For this review, take the finished solid that the model builds, in its own axes (mm). A direction names the side the tool comes from. Give positions to 0.01 mm unless a question says otherwise; leave off trailing zeros. Loops run counter-clockwise (first coordinate to the right, second up) from the corner with the lowest first, then second, coordinate; pieces in that order, holes last. Notation, with made-up numbers: (85.25, 15.25) - (124.25, 15.25) arc R8 cw to (124.25, 20.25) - close; hole circle Ø9 at (-33, 43.25). An arc over 180 degrees is marked (long way). Answer in a Markdown table with one row per item.
```python
from build123d import *

# Parameters (mm, degrees)
BOSS_EXTRUDE1_DEPTH        = 6
SKETCH2_R                  = 2.025
CUT_EXTRUDE1_DEPTH         = 68.55671766
SKETCH3_R                  = 2
CUT_EXTRUDE2_DEPTH         = 67.962004906
FILLET1_R                  = 5
M3X0_5_TAPPED_HOLE1_REACH  = 72.92
M3X0_5_TAPPED_HOLE1_BORE_R = 1.5


with BuildPart() as part:
    # Sketch1 → Boss-Extrude1 (new, symmetric)
    with BuildSketch(Plane.XY):
        Polygon((4, 0), (-23, 0), (-35, -8), (-66.211102551, -8), (-66.211102551, -4), (-36.211102551, -4), (-24.211102551, 4), (4, 4), align=None)
    extrude(amount=BOSS_EXTRUDE1_DEPTH, both=True)

    # Sketch2 → Cut-Extrude1 (cut, through all)
    with BuildSketch(Plane(origin=(0, 4, 0), x_dir=(1, 0, 0), z_dir=(0, 1, 0))):
        with Locations(Location((0, 0, 0), (0, 0, 180))):
            Circle(SKETCH2_R)
    extrude(amount=-CUT_EXTRUDE1_DEPTH, mode=Mode.SUBTRACT)

    # Sketch3 → Cut-Extrude2 (cut, through all)
    with BuildSketch(Plane(origin=(0, -4, 0), x_dir=(1, 0, 0), z_dir=(0, 1, 0))):
        with Locations(Location((-62.211102551, 0, 0), (0, 0, 270))):
            Circle(SKETCH3_R)
        with Locations(Location((-52.211102551, 2, 0), (0, 0, 270))):
            Circle(SKETCH3_R)
        with Locations(Location((-42.211102551, -2, 0), (0, 0, 270))):
            Circle(SKETCH3_R)
    extrude(amount=-CUT_EXTRUDE2_DEPTH, mode=Mode.SUBTRACT)

    # Fillet1
    fillet1_edges = [part.edges().sort_by_distance(p)[0] for p in [
        (4, 2, -6),
        (-23, 0, 0),
        (-35, -8, 0),
        (-36.211102551, -4, 0),
        (-24.211102551, 4, 0),
        (-66.211102551, -6, 6),
        (4, 2, 6),
        (-66.211102551, -6, -6),
    ]]
    fillet(fillet1_edges, radius=FILLET1_R)

    # M3x0.5 Tapped Hole1 bore → M3x0.5 Tapped Hole1 (cut, up to next)
    with BuildSketch(Plane(origin=(4, 0, 0), x_dir=(0, 0, -1), z_dir=(1, 0, 0)), mode=Mode.PRIVATE) as m3x0_5_tapped_hole1_sk1:
        with Locations((0, 2)):
            Circle(M3X0_5_TAPPED_HOLE1_BORE_R)
    m3x0_5_tapped_hole1_tool1 = extrude(m3x0_5_tapped_hole1_sk1.sketch, amount=-M3X0_5_TAPPED_HOLE1_REACH, mode=Mode.PRIVATE) & part.part
    add(m3x0_5_tapped_hole1_tool1.solids().sort_by_distance((4, 2, 0))[0], mode=Mode.SUBTRACT)


solid = part.part
```
1. Mouldability with a two-part tool opening along X and no side actions: class faces 1 (the face through (-52, -4, 1)), 2 (the face through (-29, -4, 0)), 3 (the face through (-1.93, 2.03, 0.61)) as released by +X, released by -X, zero draft, split by the parting line, or undercut.
Values:
| item | result |
|---|---|
| face 1 | zero draft |
| face 2 | released by +X |
| face 3 | undercut |
2. We need section D-D, the plane y = -1.5. Give the boundary of the cut face in (x, z).
Values:
| item | result |
|---|---|
| outline | (-32.46, -6) - (-25.25, -6) - (-25.25, 6) - (-32.46, 6) - close |
3. Wall thickness on line 1 (Y direction, x = 2.7, z = 0); line 2 (Y direction, x = -53.5, z = 1.25); line 3 (Z direction, x = 0, y = 2.3) (3 decimals): over which ranges is each line inside the solid? List them lowest first. Write a range as [from, to].
Values:
| item | result |
|---|---|
| line 1 | y = [0, 0.5], [3.5, 4] |
| line 2 | y = [-8, -4] |
| line 3 | z = [-5.899, -2.025], [2.025, 5.899] |
4. We need section C-C, the plane x = -8. Give the boundary of the cut face in (y, z).
Values:
| item | result |
|---|---|
| outline | (0, -6) - (4, -6) - (4, 6) - (0, 6) - close |
5. For faces 4 (the face through (-9, 0, 0)), 5 (the face through (3, 2, 4)), list the 3-axis set-ups (+Z, -Z, +X, -X, +Y, -Y) from which the entire face can be reached by the end or side of a thin tool; tool diameter is ignored.
Values:
| item | result |
|---|---|
| face 4 | +Z, -Z, +X, -Y |
| face 5 | +Z, +X, +Y, -Y |
6. Clearance check with flat-ended pins moving along their axes: pin 1 (1.5 mm diameter, centred on x = -36.5, z = -4.5, fed in from +Y); pin 2 (6.5 mm diameter, centred on x = 0, z = 0, fed in from -Y); pin 3 (1 mm diameter, centred on x = -58.5, y = -2.5, fed in from -Z); pin 4 (4.5 mm diameter, centred on x = -52.21, z = -2, fed in from +Y). State where each tip first meets the part, or that it passes through.
Values:
| item | result |
|---|---|
| pin 1 | stops at y = -3.59 |
| pin 2 | stops at y = 0 |
| pin 3 | passes through |
| pin 4 | stops at y = -4 |
7. We need section B-B, the plane y = -5. Give the boundary of the cut face in (x, z).
Values:
| item | result |
|---|---|
| outline | (-66.21, -1) arc R5 ccw to (-61.21, -6) - (-30.5, -6) - (-30.5, 6) - (-61.21, 6) arc R5 ccw to (-66.21, 1) - close; hole circle Ø4 at (-62.21, 0); hole circle Ø4 at (-52.21, -2); hole circle Ø4 at (-42.21, 2) |
8. We need section A-A, the plane x = 0. Give the boundary of the cut face in (y, z) (3 decimals).
Values:
| item | result |
|---|---|
| outline | (0, -5.899) - (4, -5.899) - (4, -2.025) - (0, -2.025) - close; (0, 2.025) - (4, 2.025) - (4, 5.899) - (0, 5.899) - close |
